Autodesk Inventor part; units mm, degrees
ref_plane "YZ Plane" through (0, 0, 0) normal (1, 0, 0) x (0, 1, 0)
ref_plane "XZ Plane" through (0, 0, 0) normal (0, 1, 0) x (-1, 0, 0)
ref_plane "XY Plane" through (0, 0, 0) normal (0, 0, 1) x (1, 0, 0)
sketch "Sketch1" plane through (0, 0, 0) normal (0, 0, 1) x (1, 0, 0)
  line L0 (0, 0) -> (25.4, 0)
  line L1 (25.4, 0) -> (25.4, 2.9972)
  line L2 (25.4, 2.9972) -> (0, 2.9972)
  line L3 (-355.6, 206.1972) -> (0, 2.9972)
  line L4 (-355.6, 206.1972) -> (-381, 206.1972)
  line L5 (-381, 206.1972) -> (-381, 203.2)
  line L6 (-381, 203.2) -> (-355.6, 203.2)
  line L7 (-355.6, 203.2) -> (0, 0)
  dimension "d0" = 25.4
  dimension "d1" = 2.9972
  dimension "d2" = 25.4
  dimension "d3" = 25.4
  dimension "d4" = 2.9972
  dimension "d5" = 25.4
extrude "Extrusion1" add sketch "Sketch1" along normal mid plane 279.4
properties part number "TemporaryLexan"
The listing builds one solid part. Answer for the finished solid, in the listing's coordinates (mm). A direction names the side the tool comes from. Give positions to 0.01 mm unless a question says otherwise; leave off trailing zeros. Write each loop counter-clockwise with the first axis right and the second up, starting at its lowest first coordinate (ties: lowest second). Pieces come first, ordered by that corner, then holes. Notation, with made-up numbers: (71, -24.75) -> (110, -24.75) arc R24 ccw to (110, -6.75) -> close; hole circle Ø10 at (47, 29.5). An arc over 180 degrees is marked (long way). Use a Markdown table: item, result.
(1) Section A-A, the plane z = 106.5 is taken. Determine the outline of the cut face in (x, y), then the cut area to 3 significant figures.
Return value:
| item | result |
|---|---|
| outline | (-381, 203.2) -> (-355.6, 203.2) -> (0, 0) -> (25.4, 0) -> (25.4, 3) -> (0, 3) -> (-355.6, 206.2) -> (-381, 206.2) -> close |
| area | 1,220 mm2 |
(2) Flat-ended cylindrical pins translate along their axes: P1, Ø1.5, axis at y = 157.5, z = 88.5, coming from the -X side; P2, Ø20.5, axis at x = 12, z = 61, coming from the +Y side; P3, Ø4, axis at x = -283, z = -97.5, coming from the -Y side. Find the tip coordinate at first contact, or state that the pin passes through.
Return value:
| item | result |
|---|---|
| P1 | x = -276.94 |
| P2 | y = 3 |
| P3 | y = 160.57 |
(3) Section B-B, the plane y = 50.5 is taken. Determine the outline of the cut face in (x, z) (3 decimals), then the cut area to 3 significant figures.
Return value:
| item | result |
|---|---|
| outline | (-88.375, -139.7) -> (-83.13, -139.7) -> (-83.13, 139.7) -> (-88.375, 139.7) -> close |
| area | 1,470 mm2 |
(4) Section C-C, the plane x = -161 is taken. Determine the outline of the cut face in (y, z).
Return value:
| item | result |
|---|---|
| outline | (92, -139.7) -> (95, -139.7) -> (95, 139.7) -> (92, 139.7) -> close |
(5) For faces 1 (the flat face through (-368, 203.2, -2)), 2 (the flat face through (13, 2.997, -2)), 3 (the flat face through (-368, 206.197, -2)), determine the directions among +Z, -Z, +X, -X, +Y, -Y from which every point of the face is accessible in a straight line to the end or side of a thin tool.
Return value:
| item | result |
|---|---|
| face 1 | +Z, -Z, -X, -Y |
| face 2 | +Z, -Z, +X, +Y |
| face 3 | +Z, -Z, +X, -X, +Y |
(6) Find the intervals of material crossed by probe 1 along Y at (x, z) = (1.5, 128); probe 2 along X at (y, z) = (135, 13); probe 3 along X at (y, z) = (180, -118.5), in increasing order. Write a range as from..to.
Return value:
| item | result |
|---|---|
| probe 1 | 0..3 |
| probe 2 | -236.25..-231 |
| probe 3 | -315..-309.75 |
